Model file for the job. Use its own axes, mm. A direction names the side the tool comes from. Coordinates: 2 decimals unless noted, no trailing zeros. Write each loop counter-clockwise with the first axis right and the second up, starting at its lowest first coordinate (ties: lowest second). Pieces come first, ordered by that corner, then holes. Notation, with made-up numbers: M 20.5,3 L 24.5,3 A7 ccw 24.5,14 Z; hole C 24.5,-5 d10. An arc over 180 degrees is marked long. One line per question, with ' | ' between items. Start each with the question number.
(1) Two-plate mould, pull along Y, no slides. Class faces 4 (the face through (0, 0, 0)), 5 (the face through (-5, 81.534, 5)), 6 (the face through (0.9, 85.33, 2.86)): +Y half, -Y half, draft (parallel to the pull), parting line (faces both ways), or undercut.
(2) Wall check: probe 1 along Y at (x, z) = (1.5, -7); probe 2 along Y at (x, z) = (-3.25, 2); probe 3 along Z at (x, y) = (9.25, 67.5). Give the ranges that are in metal, low to high.
(3) Cut at A-A (y = 27.5). Write the cut outline in (x, z).
(4) Tool access for faces 1 (the face through (-1, 84.074, -3)), 2 (the face through (-5.33, 82.79, 2.77)), 3 (the face through (3.3, 40.2, 10.48)): list every direction of +Z, -Z, +X, -X, +Y, -Y with a clear straight run to the whole face (end or side of a thin tool).
(5) Flat gauge pins, fed straight in: pin 1 Ø6.5 at (x, z) = (1.5, 4) entering from +Y; pin 2 Ø1.5 at (y, z) = (55.5, -7) entering from +X; pin 3 Ø1 at (x, y) = (-3.5, 21.5) entering from -Z; pin 4 Ø6 at (y, z) = (84, 7) entering from -X. Where does each tip first touch, or does it go through?
(6) Cut at B-B (x = 8.5). Write the cut outline in (y, z).
from build123d import *

# Parameters (mm, degrees)
SKETCH1_R           = 10.9855
BOSS_EXTRUDE1_DEPTH = 81.534
SKETCH2_R           = 6.0071
BOSS_EXTRUDE2_DEPTH = 2.54
SKETCH3_R           = 2.9972
BOSS_EXTRUDE3_DEPTH = 2.54
SKETCH4_R           = 4.7625
BOSS_EXTRUDE4_DEPTH = 7.62
CUT_EXTRUDE1_DEPTH  = 7.62


with BuildPart() as part:
    # Sketch1 → Boss-Extrude1 (new body)
    with BuildSketch(Plane(origin=(0, 0, 0), x_dir=(1, 0, 0), z_dir=(0, 1, 0))):
        with Locations(Location((0, 0, 0), (0, 0, 270))):
            Circle(SKETCH1_R)
    extrude(amount=BOSS_EXTRUDE1_DEPTH)

    # Sketch2 → Boss-Extrude2 (add)
    with BuildSketch(Plane(origin=(0, 81.534, 0), x_dir=(1, 0, 0), z_dir=(0, 1, 0))):
        with Locations(Location((0, 0, 0), (0, 0, 270))):
            Circle(SKETCH2_R)
    extrude(amount=BOSS_EXTRUDE2_DEPTH)

    # Sketch3 → Boss-Extrude3 (add)
    with BuildSketch(Plane(origin=(0, 84.074, 0), x_dir=(1, 0, 0), z_dir=(0, 1, 0))):
        with Locations(Location((0, 0, 0), (0, 0, 270))):
            Circle(SKETCH3_R)
    extrude(amount=BOSS_EXTRUDE3_DEPTH)

    # Sketch4 → Boss-Extrude4 (add)
    with BuildSketch(Plane(origin=(0, 86.614, 0), x_dir=(1, 0, 0), z_dir=(0, 1, 0))):
        with Locations(Location((0, 0, 0), (0, 0, 90))):
            Circle(SKETCH4_R)
    extrude(amount=BOSS_EXTRUDE4_DEPTH)

    # Sketch7 → Cut-Extrude1 (cut)
    with BuildSketch(Plane(origin=(0, 94.234, 0), x_dir=(1, 0, 0), z_dir=(0, 1, 0))):
        Polygon((-0.85725, 4.7625), (0.85725, 4.7625), (0.398425795, 3.501890859), (-0.398425795, 3.501890859), align=None)
        Polygon((1.708213051, 3.082854338), (0.972018176, 3.38779624), (1.030534117, 4.728031646), (2.614525576, 4.071920901), align=None)
        Polygon((2.757940355, 2.194481191), (2.194481191, 2.757940355), (2.761428757, 3.973763334), (3.973763334, 2.761428757), align=None)
        Polygon((3.38779624, 0.972018176), (3.082854338, 1.708213051), (4.071920901, 2.614525576), (4.728031646, 1.030534117), align=None)
        Polygon((3.501890859, -0.398425795), (3.501890859, 0.398425795), (4.7625, 0.85725), (4.7625, -0.85725), align=None)
        Polygon((3.082854338, -1.708213051), (3.38779624, -0.972018176), (4.728031646, -1.030534117), (4.071920901, -2.614525576), align=None)
        Polygon((2.194481191, -2.757940355), (2.757940355, -2.194481191), (3.973763334, -2.761428757), (2.761428757, -3.973763334), align=None)
        Polygon((0.972018176, -3.38779624), (1.708213051, -3.082854338), (2.614525576, -4.071920901), (1.030534117, -4.728031646), align=None)
        Polygon((-0.398425795, -3.501890859), (0.398425795, -3.501890859), (0.85725, -4.7625), (-0.85725, -4.7625), align=None)
        Polygon((-1.708213051, -3.082854338), (-0.972018176, -3.38779624), (-1.030534117, -4.728031646), (-2.614525576, -4.071920901), align=None)
        Polygon((-2.757940355, -2.194481191), (-2.194481191, -2.757940355), (-2.761428757, -3.973763334), (-3.973763334, -2.761428757), align=None)
        Polygon((-3.38779624, -0.972018176), (-3.082854338, -1.708213051), (-4.071920901, -2.614525576), (-4.728031646, -1.030534117), align=None)
        Polygon((-3.501890859, 0.398425795), (-3.501890859, -0.398425795), (-4.7625, -0.85725), (-4.7625, 0.85725), align=None)
        Polygon((-3.082854338, 1.708213051), (-3.38779624, 0.972018176), (-4.728031646, 1.030534117), (-4.071920901, 2.614525576), align=None)
        Polygon((-2.194481191, 2.757940355), (-2.757940355, 2.194481191), (-3.973763334, 2.761428757), (-2.761428757, 3.973763334), align=None)
        Polygon((-0.972018176, 3.38779624), (-1.708213051, 3.082854338), (-2.614525576, 4.071920901), (-1.030534117, 4.728031646), align=None)
    extrude(amount=-CUT_EXTRUDE1_DEPTH, mode=Mode.SUBTRACT)


solid = part.part
Filled in:
1) face 4: -Y half | face 5: +Y half | face 6: undercut
2) probe 1: 0 to 81.53 | probe 2: 0 to 84.07, 86.61 to 94.23 | probe 3: -5.93 to 5.93
3) outline: C 0,0 d21.97
4) face 1: none | face 2: +Y | face 3: +Y, -Y
5) pin 1: y = 94.23 | pin 2: x = 9.03 | pin 3: z = -10.57 | pin 4: x = -9.63
6) outline: M 0,-6.96 L 81.53,-6.96 L 81.53,6.96 L 0,6.96 Z
